Geometry check sheet. Reference: drawing and pictorial views, mm from the part's lowest x, y, z. A direction names the side the tool comes from. Round coordinates to 2 decimals unless told otherwise and drop trailing zeros. Write each loop counter-clockwise with the first axis right and the second up, starting at its lowest first coordinate (ties: lowest second). Pieces come first, ordered by that corner, then holes. Notation, with made-up numbers: (39.5, -26) - (57.5, -26) arc R20 cw to (57.5, 1) - close; hole circle Ø3 at (18.5, 2.25). An arc over 180 degrees is marked (long way). Use one line per item in the form item = value. Start each with the question number.
1) Draft check along Y on the marked faces 4, 5, 6 and 7. Enter one of: +Y half, -Y half, draft (parallel to the pull), parting line (faces both ways), or undercut.
2) Section check B-B (x = 6.5). Record the boundary of the cut face in (y, z).
3) Section check A-A (y = 12.25). Record the boundary of the cut face in (x, z).
4) Section check D-D (y = 6.5). Record the boundary of the cut face in (x, z), then the cut area to 3 significant figures.
5) Section check C-C (z = 0.8). Record the boundary of the cut face in (x, y).
6) Set-up check for the marked faces 1, 2 and 3: record each of +Z, -Z, +X, -X, +Y, -Y from which the full face is reachable in a straight line by a thin tool's end or side.
7) Gauge pin test, flat end, axial feed: P1, Ø1.5, axis at x = 8.5, z = 2, coming from the +Y side. Record the tip position at first contact, or that the pin passes through.
8) Scan lines: probe 1 along X at (y, z) = (5.75, 1.35); probe 2 along X at (y, z) = (10.25, 2.1); probe 3 along Y at (x, z) = (6.5, 2.45). Record each from-to range of solid material in increasing order.
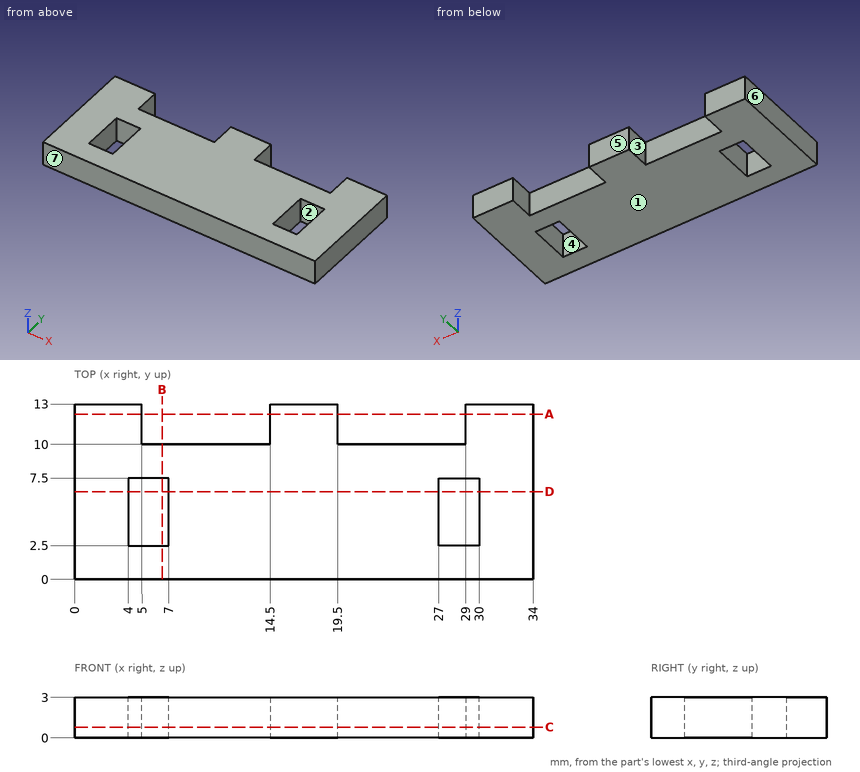
Results are:
q1.face_4 = undercut
q1.face_5 = +Y half
q1.face_6 = draft
q1.face_7 = -Y half
q2.outline = (0, 0) - (2.5, 0) - (2.5, 3) - (0, 3) - close; (7.5, 0) - (10, 0) - (10, 3) - (7.5, 3) - close
q3.outline = (0, 0) - (5, 0) - (5, 3) - (0, 3) - close; (14.5, 0) - (19.5, 0) - (19.5, 3) - (14.5, 3) - close; (29, 0) - (34, 0) - (34, 3) - (29, 3) - close
q4.outline = (0, 0) - (4, 0) - (4, 3) - (0, 3) - close; (7, 0) - (27, 0) - (27, 3) - (7, 3) - close; (30, 0) - (34, 0) - (34, 3) - (30, 3) - close
q4.area = 84.0 mm²
q5.outline = (0, 0) - (34, 0) - (34, 13) - (29, 13) - (29, 10) - (19.5, 10) - (19.5, 13) - (14.5, 13) - (14.5, 10) - (5, 10) - (5, 13) - (0, 13) - close; hole (4, 2.5) - (7, 2.5) - (7, 7.5) - (4, 7.5) - close; hole (27, 2.5) - (30, 2.5) - (30, 7.5) - (27, 7.5) - close
q6.face_1 = -Z, +X, -X, +Y, -Y
q6.face_2 = +Z, -Z
q6.face_3 = +Z, -Z, +Y
q7.P1 = 10
q8.probe_1 = 0 to 4, 7 to 27, 30 to 34
q8.probe_2 = 0 to 5, 14.5 to 19.5, 29 to 34
q8.probe_3 = 0 to 2.5, 7.5 to 10
